Geometry: see drawing. Coordinates: mm, zero at the bounding-box minimum. A direction names the side the tool comes from. Round coordinates to 2 decimals unless told otherwise and drop trailing zeros. Loops run counter-clockwise (first coordinate to the right, second up) from the corner with the lowest first, then second, coordinate; pieces in that order, holes last. Notation, with made-up numbers: M 64,12 L 113,12 A15 cw 113,30 Z; hole C 73.25,8 d8. An arc over 180 degrees is marked long. Answer as a JSON object with one key per item and string values.
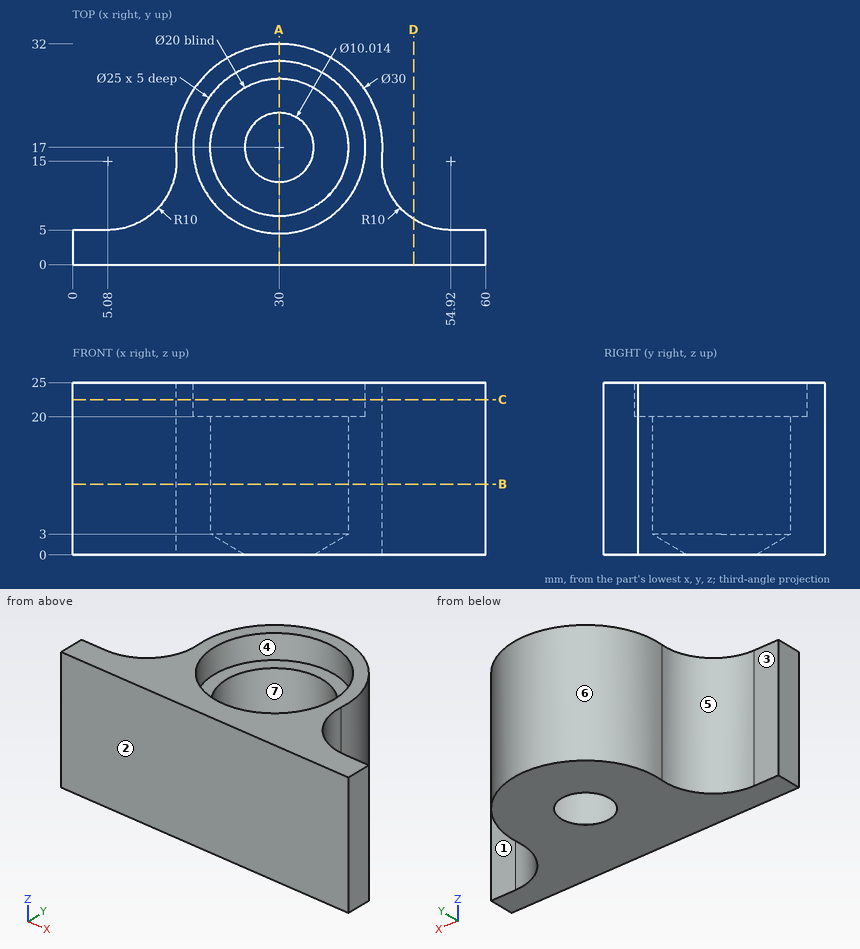
1) Section query D-D (x = 49.5). Return the cut outline in (y, z).
Results:
{"outline": "M 0,0 L 6.6,0 L 6.6,25 L 0,25 Z"}
2) Section query A-A (x = 30). Return the cut outline in (y, z).
Results:
{"outline": "M 0,0 L 11.99,0 L 7,3 L 7,20 L 4.5,20 L 4.5,25 L 0,25 Z; M 22.01,0 L 32,0 L 32,25 L 29.5,25 L 29.5,20 L 27,20 L 27,3 Z"}
3) Section query C-C (z = 22.5). Return the cut outline in (x, y), and give its area (3 significant figures).
Results:
{"outline": "M 0,0 L 60,0 L 60,5 L 54.92,5 A10 cw 44.95,15.8 A15 ccw long 15.05,15.8 A10 cw 5.08,5 L 0,5 Z; hole C 30,17 d25", "area": "564 mm2"}
4) Pin query (flat end, axial travel): P1, Ø6, axis at x = 26, y = 9.5, coming from the -Z side; P2, Ø1.5, axis at x = 57.5, z = 15, coming from the +Y side; P3, Ø1.5, axis at y = 24, z = 21.5, coming from the +X side; P4, Ø2, axis at y = 24.5, z = 2.5, coming from the +X side. Return the tip coordinate at first contact, or that it passes through.
Results:
{"P1": "z = 0", "P2": "y = 5", "P3": "x = 43.64", "P4": "x = 43.52"}
5) Ray query, line 1 (X direction, y = 17, z = 16.5); line 2 (Y direction, x = 30, z = 11.25); line 3 (Y direction, x = 30, z = 21.9). Return the intervals inside material, ascending.
Results:
{"line 1": "15 to 20, 40 to 45", "line 2": "0 to 7, 27 to 32", "line 3": "0 to 4.5, 29.5 to 32"}
6) Reachability of the marked faces 1, 2 and 3 from +Z, -Z, +X, -X, +Y, -Y: full face, straight path, thin tool, end or side. Return the list, or none.
Results:
{"face 1": "+Z, -Z, +X, +Y", "face 2": "+Z, -Z, +X, -X, -Y", "face 3": "+Z, -Z, -X, +Y"}
7) Section query B-B (z = 10.25). Return the cut outline in (x, y).
Results:
{"outline": "M 0,0 L 60,0 L 60,5 L 54.92,5 A10 cw 44.95,15.8 A15 ccw long 15.05,15.8 A10 cw 5.08,5 L 0,5 Z; hole C 30,17 d20"}
8) Pull-direction query (X, two-part tool) for the marked faces 4, 5, 6 and 7; classes: +X half, -X half, draft (parallel to the pull), parting line (faces both ways), or undercut.
Results:
{"face 4": "undercut", "face 5": "-X half", "face 6": "parting line", "face 7": "undercut"}
